Autodesk Inventor part; units mm, degrees
ref_plane "IP_DUMMY_XY" through (0, 0, 0) normal (0, 1, 0) x (1, 0, 0)
ref_plane "IP_DUMMY_YZ" through (0, 0, 0) normal (1, 0, 0) x (0, 0, -1)
ref_plane "IP_DUMMY_ZX" through (0, 0, 0) normal (0, 0, -1) x (0, 1, 0)
sketch "Sketch_1" plane through (0, 0, 0) normal (0, 0, 1) x (1, 0, 0)
  line L0 (0, 0) -> (0, 5.5)
  line L1 (0, 5.5) -> (5.25, 5.5)
  line L2 (5.25, 5.5) -> (5.25, 4)
  line L3 (5.25, 4) -> (5.9, 4)
  line L4 (5.9, 4) -> (7.5, 3.0762)
  line L5 (7.5, 3.0762) -> (7.5, 0.9238)
  line L6 (7.5, 0.9238) -> (5.9, 0)
  line L7 (5.9, 0) -> (0, 0)
  line L8 (0, 0) -> (0, 5.5)
revolve "Revolution1" add sketch "Sketch_1" angle 360 about axis through (0, 0, 0) along (0, -1, 0)
sketch "Sketch_2" plane through (0, 0, 0) normal (0, 1, 0) x (-1, 0, 0)
  line L0 (17.2177, 15.6183) -> (-16.6532, 15.6183)
  line L1 (-16.6532, 15.6183) -> (-16.6532, -14.1129)
  line L2 (-16.6532, -14.1129) -> (17.2177, -14.1129)
  line L3 (17.2177, -14.1129) -> (17.2177, 15.6183)
  line L4 (6.9282, 0) -> (3.4641, 6)
  line L5 (3.4641, 6) -> (-3.4641, 6)
  line L6 (-3.4641, 6) -> (-6.9282, 0)
  line L7 (-6.9282, 0) -> (-3.4641, -6)
  line L8 (-3.4641, -6) -> (3.4641, -6)
  line L9 (3.4641, -6) -> (6.9282, 0)
extrude "Extrusion1" cut sketch "Sketch_2" along normal blind 4
sketch "Sketch_3" plane through (0, 0, 0) normal (0, 0, 1) x (1, 0, 0)
  line L0 (0, 5.5) -> (0, 26.1)
  line L1 (0, 26.1) -> (4.7, 26.1)
  arc A0 (4.9, 25.9) -> (4.7, 26.1) centre (4.7, 25.9) ccw
  line L2 (4.9, 25.9) -> (4.9, 24.9)
  line L3 (4.9, 24.9) -> (3.5, 24.9)
  line L4 (3.5, 24.9) -> (3.5, 24)
  line L5 (3.5, 24) -> (4.8, 24)
  line L6 (4.8, 24) -> (4.934, 23.5)
  line L7 (4.934, 23.5) -> (5.4, 23.2309)
  line L8 (5.4, 23.2309) -> (5.4, 22.5)
  line L9 (5.4, 22.5) -> (5.5, 22.5)
  line L10 (5.5, 22.5) -> (6, 22)
  line L11 (6, 22) -> (6, 6.25)
  line L12 (6, 6.25) -> (5.25, 5.5)
  line L13 (5.25, 5.5) -> (0, 5.5)
  line L14 (0, 5.5) -> (0, 26.1)
revolve "Revolution2" add sketch "Sketch_3" angle 360 about axis through (0, 5.5, 0) along (0, -1, 0)
thread "Thread1"
sketch "Sketch_4" plane through (0, 0, 0) normal (0, 0, 1) x (1, 0, 0)
  line L0 (0, 14.4) -> (0, 26.1)
  line L1 (0, 26.1) -> (3, 26.1)
  line L2 (3, 26.1) -> (3, 14.4)
  line L3 (3, 14.4) -> (0, 14.4)
  line L4 (0, 14.4) -> (0, 26.1)
revolve "Revolution3" cut sketch "Sketch_4" angle 360 about axis through (0, 14.4, 0) along (0, -1, 0)
sketch "Sketch_5" plane through (0, 0, 0) normal (0, 0, 1) x (1, 0, 0)
  line L0 (0, 0) -> (0, 6.25)
  line L1 (0, 6.25) -> (1.621, 6.25)
  line L2 (1.621, 6.25) -> (1.621, 0)
  line L3 (1.621, 0) -> (0, 0)
  line L4 (0, 0) -> (0, 6.25)
revolve "Revolution4" cut sketch "Sketch_5" angle 360 about axis through (0, 0, 0) along (0, -1, 0)
thread "Thread2"
ref_plane "IP_DUMMY_XY" through (0, 0, 0) normal (0, 1, 0) x (1, 0, 0)
ref_plane "IP_DUMMY_YZ" through (0, 0, 0) normal (1, 0, 0) x (0, 0, -1)
ref_plane "IP_DUMMY_ZX" through (0, 0, 0) normal (0, 0, -1) x (0, 1, 0)
ref_plane "IP_NUT1_XY" through (0, 11, 0) normal (0, 1, 0) x (1, 0, 0)
ref_plane "IP_NUT1_YZ" through (0, 11, 0) normal (1, 0, 0) x (0, 0, -1)
ref_plane "IP_NUT1_ZX" through (0, 11, 0) normal (0, 0, -1) x (0, 1, 0)
ref_plane "IP_NUT2_XY" through (0, 17, 0) normal (0, 1, 0) x (1, 0, 0)
ref_plane "IP_NUT2_YZ" through (0, 17, 0) normal (1, 0, 0) x (0, 0, -1)
ref_plane "IP_NUT2_ZX" through (0, 17, 0) normal (0, 0, -1) x (0, 1, 0)
properties part number "FVPA106J"
Input: part model. Units: mm. Frame: model coordinates. A direction names the side the tool comes from. Coordinates: 2 decimals unless noted, no trailing zeros. Loops run counter-clockwise (first coordinate to the right, second up) from the corner with the lowest first, then second, coordinate; pieces in that order, holes last. Notation, with made-up numbers: M 60,-37 L 73,-37 A22 ccw 73,-28 Z; hole C 25,10 d8. An arc over 180 degrees is marked long. Use a Markdown table: item, result. Add a question column.
1) Set-up query: faces 4 (the cylindrical face through (3.233, 24.444, -1.341)), 5 (the cylindrical face through (-6, 14, 0)), 6 (the flat face through (0, 6.25, 0)). Return all of +Z, -Z, +X, -X, +Y, -Y with unobstructed straight access to the full face (end or side cutting, diameter ignored); none if empty.
2) Draft query along X for faces 1 (the flat face through (2.1, 24.9, -3.2)), 2 (the flat face through (-5.172, 1.973, -3.042)), 3 (the cylindrical face through (0.748, 3.081, -1.438)). Return one class per face: +X half, -X half, draft (parallel to the pull), parting line (faces both ways), or undercut.
3) Section C-C, the plane y = 17.5. Return the cut outline in (x, z).
4) Section B-B, the plane y = 13. Return the cut outline in (x, z).
5) Section A-A, the plane y = 1.5. Return the cut outline in (x, z).
6) Line query: L1, parallel to Y at x = 3.75, z = -0.5; L2, parallel to Z at x = 0, y = 21.75; L3, parallel to Z at x = 0, y = 3.75. Output: solid intervals per line, ascending. Write a range as from..to.
7) Pin query (flat end, axial travel): P1, Ø1, axis at y = 5.5, z = 4.5, coming from the +X side; P2, Ø2, axis at x = 4.5, y = 8.5, coming from the +Z side; P3, Ø5, axis at x = 0, z = 0, coming from the +Y side. Return the tip coordinate at first contact, or that it passes through.
Answer below:
| question | item | result |
|---|---|---|
| 1 | face 4 | none |
| 1 | face 5 | +Y |
| 1 | face 6 | -Y |
| 2 | face 1 | draft |
| 2 | face 2 | -X half |
| 2 | face 3 | undercut |
| 3 | outline | C 0,0 d12; hole C 0,0 d6 |
| 4 | outline | C 0,0 d12 |
| 5 | outline | M -6.93,0 L -3.46,-6 L 3.46,-6 L 6.93,0 L 3.46,6 L -3.46,6 Z; hole C 0,0 d3.24 |
| 6 | L1 | 0..24, 24.9..26.1 |
| 6 | L2 | -6..-3, 3..6 |
| 6 | L3 | -6..-1.62, 1.62..6 |
| 7 | P1 | x = 3.78 |
| 7 | P2 | z = 4.87 |
| 7 | P3 | y = 14.4 |
